Geometry: final body of the model. Coordinates: model frame, mm. Give positions to 0.01 mm unless a question says otherwise; leave off trailing zeros. Loops run counter-clockwise (first coordinate to the right, second up) from the corner with the lowest first, then second, coordinate; pieces in that order, holes last. Notation, with made-up numbers: (84.25, -36.5) -> (117.25, -36.5) arc R16 cw to (117.25, -8.5) -> close; hole circle Ø2 at (-2.75, 42.25). An arc over 180 degrees is marked (long way). Answer in a Markdown table with one row per item. Add a question column.
1) First-contact query: P1, Ø3, axis at x = -46.482, y = -12.7, coming from the +Z side. Flat tip, straight axial feed; report the tip coordinate or a pass-through.
2) Draft query along X for faces 1 (the cylindrical face through (-45.9, -20.18, 0.88)), 2 (the flat face through (-22, 1, 1.978)), 3 (the cylindrical face through (-46.62, -11.63, 0.88)), 4 (the flat face through (50.201, -38.424, 0.877)). Return one class per face: +X half, -X half, draft (parallel to the pull), parting line (faces both ways), or undercut.
3) Section query B-B (y = 12.7). Give the number of separate pieces and of enclosed holes in the cut face, plus the area to 3 significant figures.
4) Section query D-D (y = -34). Return the cut outline in (x, z) (3 decimals), plus the area to 3 significant figures.
5) Section query A-A (x = 44.45). Return the cut outline in (y, z), plus the area to 3 significant figures.
6) Line query: line 1 (Y direction, x = 44.45, z = 1.35); line 2 (X direction, y = -18.5, z = 1.85) (3 decimals); line 3 (Z direction, x = -48, y = 7). Output: solid intervals per line, ascending. Write a range as from..to.
7) Section query C-C (y = -19.05). Return the cut outline in (x, z) (3 decimals), plus the area to 3 significant figures.
```python
from build123d import *

# Parameters (mm, degrees)
SKETCH1_W           = 105.41
SKETCH1_H           = 82
SKETCH1_R           = 1.0795
SKETCH1_R_2         = 1.27
BOSS_EXTRUDE1_DEPTH = 1.778
BOSS_EXTRUDE2_DEPTH = 0.2
CHAMFER2_SIZE       = 5.08


with BuildPart() as part:
    # Sketch1 → Boss-Extrude1 (new body)
    with BuildSketch(Plane.XY):
        Rectangle(SKETCH1_W, SKETCH1_H)
        with Locations((44.45, 12.7)):
            Circle(SKETCH1_R, mode=Mode.SUBTRACT)
        with Locations((44.45, -12.7)):
            Circle(SKETCH1_R, mode=Mode.SUBTRACT)
        with Locations((-46.482, 12.7)):
            Circle(SKETCH1_R, mode=Mode.SUBTRACT)
        with Locations((-46.482, -12.7)):
            Circle(SKETCH1_R, mode=Mode.SUBTRACT)
        with Locations((-46.482, -19.05)):
            Circle(SKETCH1_R_2, mode=Mode.SUBTRACT)
    extrude(amount=BOSS_EXTRUDE1_DEPTH)

    # Sketch2 → Boss-Extrude2 (add)
    with BuildSketch(Plane.XY.offset(1.778)):
        Polygon((-11, 39.095), (-1, 29.095), (-1, -29.095), (-11, -39.095), (-42.705, -39.095), (-42.705, 39.095), align=None)
        Polygon((42.705, 20.205), (38.895, 16.395), (38.895, -16.395), (42.705, -20.205), (42.705, -29.095), (32.705, -39.095), (1, -39.095), (1, 39.095), (32.705, 39.095), (42.705, 29.095), align=None)
    extrude(amount=BOSS_EXTRUDE2_DEPTH)

    # Chamfer2
    chamfer2_edges = [part.edges().sort_by_distance(p)[0] for p in [
        (52.705, 41, 0.889),
        (52.705, -41, 0.889),
    ]]
    chamfer(chamfer2_edges, length=CHAMFER2_SIZE)


solid = part.part
```
Evaluation:
| question | item | result |
|---|---|---|
| 1 | P1 | z = 1.78 |
| 2 | face 1 | undercut |
| 2 | face 2 | draft |
| 2 | face 3 | undercut |
| 2 | face 4 | +X half |
| 3 | separate pieces | 3 |
| 3 | enclosed holes | 0 |
| 3 | area | 196 mm² |
| 4 | outline | (-52.705, 0) -> (52.705, 0) -> (52.705, 1.778) -> (37.8, 1.778) -> (37.8, 1.978) -> (1, 1.978) -> (1, 1.778) -> (-5.905, 1.778) -> (-5.905, 1.978) -> (-42.705, 1.978) -> (-42.705, 1.778) -> (-52.705, 1.778) -> close |
| 4 | area | 202 mm² |
| 5 | outline | (-41, 0) -> (-13.78, 0) -> (-13.78, 1.78) -> (-41, 1.78) -> close; (-11.62, 0) -> (11.62, 0) -> (11.62, 1.78) -> (-11.62, 1.78) -> close; (13.78, 0) -> (41, 0) -> (41, 1.78) -> (13.78, 1.78) -> close |
| 5 | area | 138 mm² |
| 6 | line 1 | -41..-13.78, -11.62..11.62, 13.78..41 |
| 6 | line 2 | -42.705..-1, 1..41 |
| 6 | line 3 | 0..1.78 |
| 7 | outline | (-52.705, 0) -> (-47.752, 0) -> (-47.752, 1.778) -> (-52.705, 1.778) -> close; (-45.212, 0) -> (52.705, 0) -> (52.705, 1.778) -> (41.55, 1.778) -> (41.55, 1.978) -> (1, 1.978) -> (1, 1.778) -> (-1, 1.778) -> (-1, 1.978) -> (-42.705, 1.978) -> (-42.705, 1.778) -> (-45.212, 1.778) -> close |
| 7 | area | 199 mm² |
